Here's how the part is built. I have some questions about the finished solid (model axes, mm). A direction names the side the tool comes from. Round coordinates to 2 decimals unless told otherwise and drop trailing zeros. Order: outer loops, then holes, each group sorted by start corner. A loop starts at its lowest first (then second) coordinate and runs counter-clockwise, first axis right, second up. Notation, with made-up numbers: (56.25, 69) -> (112.25, 69) arc R19 cw to (112.25, 91) -> close; hole circle Ø3 at (8.5, 88.5). An arc over 180 degrees is marked (long way). Use a Markdown table: item, result. Add a question column.
(1) I want a section at C-C, the plane y = -100. Please give me the cut outline in (x, z), then the cut area to 3 significant figures.
(2) I'm going to push flat-ended pins straight in: P1, Ø1.5, axis at x = 1, z = 5, coming from the +Y side; P2, Ø1.5, axis at x = 2, z = 7.5, coming from the -Y side; P3, Ø1, axis at x = 1.5, z = -24.5, coming from the +Y side. Where does each tip first touch, or does it pass through?
(3) On a 3-axis mill with a long thin cutter (end or side, diameter ignored), from which of +Z, -Z, +X, -X, +Y, -Y can I reach the whole of each face in a straight line? I mean faces 5 (the face through (1.48, -119.99, 0.97)), 6 (the face through (1, -62, 25)). Say none if no direction works.
(4) I want a section at B-B, the plane y = -21.5. Please give me the cut outline in (x, z).
(5) Thinking about a two-plate mould opening in Z: for faces 1 (the face through (0, -37, 1)), 2 (the face through (1, -62, -25)), 3 (the face through (1.48, 43.99, -0.97)), 4 (the face through (1, -37, 44)), which applies, pulls with the +Z half, pulls with the -Z half, needs draft (parallel to the pull), parting line crosses it, or undercut?
(6) I want a section at D-D, the plane z = 14.5. Please give me the cut outline in (x, y), then the cut area to 3 significant figures.
(7) If I drill on probe 1 along Y at (x, z) = (1.1, 0); probe 2 along Y at (x, z) = (2.85, -8.5); probe 3 along Y at (x, z) = (1.1, -6.5), over which ranges is the centre line in solid material (lowest first)?
(8) I want a section at A-A, the plane x = 2.3. Please give me the cut outline in (y, z).
from build123d import *

# Parameters (mm, degrees)
SKETCH1_R           = 1.5
SKETCH1_R_2         = 4
SKETCH1_W           = 50
SKETCH1_H           = 3
BOSS_EXTRUDE1_DEPTH = 3


with BuildPart() as part:
    # Sketch1 → Boss-Extrude1 (new body)
    with BuildSketch(Plane(origin=(0, 0, 0), x_dir=(0, 0, -1), z_dir=(1, 0, 0))):
        with BuildLine():
            Line((-44, 0), (-44, -76))
            ThreePointArc((-44, -76), (0, -120), (44, -76))
            Line((44, -76), (44, 0))
            ThreePointArc((44, 0), (0, 44), (-44, 0))
        make_face()
        with Locations((0, -21.5)):
            Circle(SKETCH1_R, mode=Mode.SUBTRACT)
        with Locations((0, -71.5)):
            Circle(SKETCH1_R, mode=Mode.SUBTRACT)
        with Locations((0, -100)):
            Circle(SKETCH1_R_2, mode=Mode.SUBTRACT)
        with Locations((-8.5, -100)):
            Circle(SKETCH1_R, mode=Mode.SUBTRACT)
        with Locations((8.5, -100)):
            Circle(SKETCH1_R, mode=Mode.SUBTRACT)
        with Locations((0, -11.5)):
            Rectangle(SKETCH1_W, SKETCH1_H, mode=Mode.SUBTRACT)
        with Locations((0, -61.5)):
            Rectangle(SKETCH1_W, SKETCH1_H, mode=Mode.SUBTRACT)
    extrude(amount=BOSS_EXTRUDE1_DEPTH)


solid = part.part
Taken from the geometry:
| question | item | result |
|---|---|---|
| 1 | outline | (0, -36.88) -> (3, -36.88) -> (3, -10) -> (0, -10) -> close; (0, -7) -> (3, -7) -> (3, -4) -> (0, -4) -> close; (0, 4) -> (3, 4) -> (3, 7) -> (0, 7) -> close; (0, 10) -> (3, 10) -> (3, 36.88) -> (0, 36.88) -> close |
| 1 | area | 179 mm2 |
| 2 | P1 | stops at y = 43.79 |
| 2 | P2 | stops at y = -119.48 |
| 2 | P3 | stops at y = 36.88 |
| 3 | face 5 | +X, -X, -Y |
| 3 | face 6 | +X, -X |
| 4 | outline | (0, -44) -> (3, -44) -> (3, -1.5) -> (0, -1.5) -> close; (0, 1.5) -> (3, 1.5) -> (3, 44) -> (0, 44) -> close |
| 5 | face 1 | needs draft |
| 5 | face 2 | undercut |
| 5 | face 3 | parting line crosses it |
| 5 | face 4 | pulls with the +Z half |
| 6 | outline | (0, -117.54) -> (3, -117.54) -> (3, -63) -> (0, -63) -> close; (0, -60) -> (3, -60) -> (3, -13) -> (0, -13) -> close; (0, -10) -> (3, -10) -> (3, 41.54) -> (0, 41.54) -> close |
| 6 | area | 459 mm2 |
| 7 | probe 1 | y = -120 to -104, -96 to -73, -70 to -63, -60 to -23, -20 to -13, -10 to 44 |
| 7 | probe 2 | y = -119.17 to -101.5, -98.5 to -63, -60 to -13, -10 to 43.17 |
| 7 | probe 3 | y = -119.52 to -63, -60 to -13, -10 to 43.52 |
| 8 | outline | (-76, -44) -> (0, -44) arc R44 ccw to (0, 44) -> (-76, 44) arc R44 ccw to start; hole circle Ø8 at (-100, 0); hole circle Ø3 at (-100, -8.5); hole circle Ø3 at (-100, 8.5); hole circle Ø3 at (-71.5, 0); hole (-63, -25) -> (-60, -25) -> (-60, 25) -> (-63, 25) -> close; hole circle Ø3 at (-21.5, 0); hole (-13, -25) -> (-10, -25) -> (-10, 25) -> (-13, 25) -> close |
